The model under review builds one solid part; all positions refer to its coordinate system, in mm. A direction names the side the tool comes from. Round coordinates to 2 decimals unless told otherwise and drop trailing zeros. Loops run counter-clockwise (first coordinate to the right, second up) from the corner with the lowest first, then second, coordinate; pieces in that order, holes last. Notation, with made-up numbers: M -28,10.25 L 21,10.25 A24 ccw 21,26.25 Z; hole C 37.5,55.5 d6. An arc over 180 degrees is marked long. Answer as a JSON object with one key per item and string values. Group by question number.
Item 1: Tool access review of faces 5 (the face through (1, 77, -1)), 6 (the face through (108, -74, 0)): name each direction out of +Z, -Z, +X, -X, +Y, -Y from which nothing blocks a thin tool from reaching the whole face with its end or side.
Item 2: Consider section D-D (y = -23.5). Give the boundary of the cut face in (x, z), and give its area (3 significant figures).
Item 3: Consider section C-C (z = 11). Give the boundary of the cut face in (x, y).
Item 4: Insertion check: P1, Ø1.5, axis at x = 51, y = 12, coming from the +Z side. The pin has a flat end and moves straight along its axis. Give the tip position at first contact, or say it passes through.
Item 5: The part is to be moulded in two halves that separate along Z. For faces 1 (the face through (-2, 1, -32)), 2 (the face through (-111.01, 1.08, -4.88)), 3 (the face through (110, 74.9, -0.6)), 4 (the face through (-2, 1, -30)), say which applies: +Z half, -Z half, draft (parallel to the pull), parting line (faces both ways), or undercut.
Item 6: Consider section B-B (x = 30). Give the boundary of the cut face in (y, z).
Item 7: Consider section A-A (y = 0). Give the boundary of the cut face in (x, z), and give its area (3 significant figures).
Item 8: To check wall thickness, follow line 1 (Y direction, x = 17.5, z = 14.5); line 2 (X direction, y = 9, z = -28.5); line 3 (Z direction, x = -111.2, y = 0). State the ranges of each line that lie inside material, in increasing order.
```python
from build123d import *

# Parameters (mm, degrees)
BOSS_EXTRUDE1_DEPTH = 30
SHELL1_T            = 2
SKETCH2_R           = 5
CUT_EXTRUDE1_DEPTH  = 50


with BuildPart() as part:
    # Sketch1 → Boss-Extrude1 (new, symmetric)
    with BuildSketch(Plane.XY):
        with BuildLine():
            Line((-105, -75), (105, -75))
            ThreePointArc((105, -75), (108.535533906, -73.535533906), (110, -70))
            Line((110, -70), (110, 70))
            ThreePointArc((110, 70), (108.535533906, 73.535533906), (105, 75))
            Line((105, 75), (-105, 75))
            ThreePointArc((-105, 75), (-108.535533906, 73.535533906), (-110, 70))
            Line((-110, 70), (-110, -70))
            ThreePointArc((-110, -70), (-108.535533906, -73.535533906), (-105, -75))
        make_face()
    extrude(amount=BOSS_EXTRUDE1_DEPTH, both=True)

    # Shell1
    shell1_openings = [part.faces().sort_by_distance(p)[0] for p in [
        (0, 0, 30),
    ]]
    offset(amount=SHELL1_T, openings=shell1_openings, kind=Kind.INTERSECTION)

    # Sketch2 → Cut-Extrude1 (cut)
    with BuildSketch(Plane.ZY.offset(112)):
        with Locations(Location((0, 0, 0), (0, 0, 270))):
            Circle(SKETCH2_R)
    extrude(amount=-CUT_EXTRUDE1_DEPTH, mode=Mode.SUBTRACT)


solid = part.part
```
Geometry results:
{
 "1": {"face 5": "+Z, -Z, +X, -X, +Y", "face 6": "+Z"},
 "2": {"outline": "M -112,-32 L 112,-32 L 112,30 L 110,30 L 110,-30 L -110,-30 L -110,30 L -112,30 Z", "area": "688 mm^2"},
 "3": {"outline": "M -112,-70 A7 ccw -105,-77 L 105,-77 A7 ccw 112,-70 L 112,70 A7 ccw 105,77 L -105,77 A7 ccw -112,70 Z; hole M -110,-70 A5 ccw -105,-75 L 105,-75 A5 ccw 110,-70 L 110,70 A5 ccw 105,75 L -105,75 A5 ccw -110,70 Z"},
 "4": {"P1": "stops at z = -30"},
 "5": {"face 1": "-Z half", "face 2": "undercut", "face 3": "draft", "face 4": "+Z half"},
 "6": {"outline": "M -77,-32 L 77,-32 L 77,30 L 75,30 L 75,-30 L -75,-30 L -75,30 L -77,30 Z"},
 "7": {"outline": "M -112,-32 L 112,-32 L 112,30 L 110,30 L 110,-30 L -110,-30 L -110,-5 L -112,-5 Z; M -112,5 L -110,5 L -110,30 L -112,30 Z", "area": "668 mm^2"},
 "8": {"line 1": "y = -77 to -75, 75 to 77", "line 2": "x = -112 to -110, 110 to 112", "line 3": "z = -32 to -5, 5 to 30"}
}
